Read the model definition and answer for the solid it produces. Units are mm, in the model's axes. Face numbers are marked on the shaded views. A direction names the side the tool comes from. Round coordinates to 2 decimals unless told otherwise and drop trailing zeros. Write each loop counter-clockwise with the first axis right and the second up, starting at its lowest first coordinate (ties: lowest second). Pieces come first, ordered by that corner, then holes. Notation, with made-up numbers: (79, 73) - (135, 73) arc R11 ccw to (135, 79) - close; hole circle Ø1 at (-34, 34). An arc over 180 degrees is marked (long way). Use one line per item in the form item = value. Start each with the question number.
1) For a pull along Z with two mould halves and no side action, classify the marked faces 1, 2 and 3 as released by +Z, released by -Z, zero draft, split by the parting line, or undercut.
2) The part is cut by section B-B, the plane x = -5.5. Give the vertices of the cut face in (y, z), plus the area to 3 significant figures.
3) The part is cut by section C-C, the plane y = -5.25. Count the separate pieces of the cut face and the enclosed holes in it, plus the area to 3 significant figures.
4) The part is cut by section A-A, the plane y = 7.25. Give the vertices of the cut face in (x, z).
5) Each of these flat-tipped pins is pushed along its axis until it touches: pin 1 (1.9 mm diameter, centred on y = -7.4, z = 4.28, fed in from +X); pin 2 (5 mm diameter, centred on x = -1.5, y = -3.5, fed in from -Z); pin 3 (3 mm diameter, centred on x = -12, z = 1, fed in from +Y). Where does it stop, or does it pass through?
6) Consider line 1 along X through (y, z) = (4.75, 2); line 2 along X through (y, z) = (-5.75, 1); line 3 along Y through (x, z) = (-4.25, -2.5). Determine where each line is inside the solid, lowest interval first. Write a range as from..to.
7) For the marked faces 4, 5, 6 and 7, determine the directions among +Z, -Z, +X, -X, +Y, -Y from which every point of the face is accessible in a straight line to the end or side of a thin tool.
from build123d import *

# Parameters (mm, degrees)
F4_DEPTH = 1.3
F6_DEPTH = 1.05
F5_R     = 0.725
F7_DEPTH = 0.67
F8_R     = 0.3621320344
F8_2_R   = 0.3621320344


# Not quite as in the source:
# - a fillet or chamfer that OpenCascade refuses, or shapes differently, is made with other operations: its cross-section is extruded or revolved along the edge and cut away or added


with BuildPart() as f1:
    # F0 (on Front) → F1 (revolve)
    with BuildSketch(Plane.XZ):
        Polygon((-8.85, 2), (-8.85, 0.75), (-2.35, 0.75), (-2.35, 6.5), (-7.85, 6.5), (-7.85, 2), align=None)
    revolve(axis=Axis((6.5496404592, 0, 0), (1, 0, 0)))

    # F3: chamfer of 2 x 1 on 1 edges, made by hand

    # F3_s1 → F3_t2 (revolve, cut)
    with BuildSketch(Plane.XZ):
        Polygon((-6.85, 6.5), (-7.85, 4.5), (-7.85, 6.5), align=None)
    revolve(axis=Axis((-7.85, 0, 0), (1, 0, 0)), mode=Mode.SUBTRACT)

    # F2 (on face) → F4 (cut)
    with BuildSketch(Plane(origin=(-7.85, 0, 0), x_dir=(0, -1, 0), z_dir=(-1, 0, 0))):
        with BuildLine():
            Line((-1.65, 2.2843407316), (-1.65, 6.2870899469))
            ThreePointArc((-1.65, 6.2870899469), (-5.6291651246, 3.25), (-6.2697796099, -1.7146030572))
            Line((-6.2697796099, -1.7146030572), (-2.8032971045, 0.2867715504))
            ThreePointArc((-2.8032971045, 0.2867715504), (-1.9590250278, 1.1310436271), (-1.65, 2.2843407316))
        make_face()
        with BuildLine():
            ThreePointArc((6.5, 0), (5.14660082, 3.9702015062), (1.65, 6.2870899469))
            Line((1.65, 6.2870899469), (1.65, 2.2843407316))
            ThreePointArc((1.65, 2.2843407316), (1.9590250278, 1.1310436271), (2.8032971045, 0.2867715504))
            Line((2.8032971045, 0.2867715504), (6.2697796099, -1.7146030572))
            ThreePointArc((6.2697796099, -1.7146030572), (6.4421878063, -0.8649949526), (6.5, 0))
        make_face()
        with BuildLine():
            Line((-1.1532971045, -2.571112282), (-4.6197796099, -4.5724868897))
            ThreePointArc((-4.6197796099, -4.5724868897), (0, -6.5), (4.6197796099, -4.5724868897))
            Line((4.6197796099, -4.5724868897), (1.1532971045, -2.571112282))
            ThreePointArc((1.1532971045, -2.571112282), (0, -2.2620872543), (-1.1532971045, -2.571112282))
        make_face()
    extrude(amount=-F4_DEPTH, mode=Mode.SUBTRACT)

    # F8
    f8_edges = [f1.edges().sort_by_distance(p)[0] for p in [
        (-7.85, 0, 4.5),
        (-7.85, 3.897114, -2.25),
        (-7.85, -3.897114, -2.25),
        (-8.85, 0, -2),
    ]]
    fillet(f8_edges, radius=F8_R)



with BuildPart() as f1b:
    # F0 (on Front) → F1, piece 2 (revolve)
    with BuildSketch(Plane.XZ):
        Polygon((-0.67, 0.75), (0, 0.75), (0, 6.2), (-1.05, 6.2), (-1.55, 6.5), (-2.05, 6.5), (-2.05, 5.64), (-0.67, 5.64), align=None)
    revolve(axis=Axis((6.5496404592, 0, 0), (1, 0, 0)))

    # F5 (on face) → F6 (cut)
    with BuildSketch(Plane.YZ):
        with BuildLine():
            ThreePointArc((4.3433258161, 4.4244232228), (0, 6.2), (-4.3433258161, 4.4244232228))
            Line((-4.3433258161, 4.4244232228), (-1.1869283577, 2.6020763005))
            ThreePointArc((-1.1869283577, 2.6020763005), (0, 2.86), (1.1869283577, 2.6020763005))
            Line((1.1869283577, 2.6020763005), (4.3433258161, 4.4244232228))
        make_face()
        with BuildLine():
            Line((1.66, -2.3289482605), (1.66, -5.9736421051))
            ThreePointArc((1.66, -5.9736421051), (4.936192865, -3.75153302), (6.2, 0))
            ThreePointArc((6.2, 0), (6.150634929, 0.780826466), (6.0033258161, 1.5492188823))
            Line((6.0033258161, 1.5492188823), (2.8469283577, -0.27312804))
            ThreePointArc((2.8469283577, -0.27312804), (2.4768326548, -1.43), (1.66, -2.3289482605))
        make_face()
        with BuildLine():
            ThreePointArc((-6.0033258161, 1.5492188823), (-5.3693575035, -3.1), (-1.66, -5.9736421051))
            Line((-1.66, -5.9736421051), (-1.66, -2.3289482605))
            ThreePointArc((-1.66, -2.3289482605), (-2.4768326548, -1.43), (-2.8469283577, -0.27312804))
            Line((-2.8469283577, -0.27312804), (-6.0033258161, 1.5492188823))
        make_face()
    extrude(amount=-F6_DEPTH, mode=Mode.SUBTRACT)

    # F5 (on face) → F7 (join)
    with BuildSketch(Plane.YZ):
        with BuildLine():
            Line((-8.2345172024, 2.8373978297), (-6.0033258161, 1.5492188823))
            ThreePointArc((-6.0033258161, 1.5492188823), (-5.3693575035, 3.1), (-4.3433258161, 4.4244232228))
            Line((-4.3433258161, 4.4244232228), (-6.5745172024, 5.7126021703))
            ThreePointArc((-6.5745172024, 5.7126021703), (-8.8421193726, 5.105), (-8.2345172024, 2.8373978297))
        make_face()
        with Locations((-7.4045172024, 4.275)):
            Circle(F5_R, mode=Mode.SUBTRACT)
        with BuildLine():
            ThreePointArc((4.3433258161, 4.4244232228), (5.3693575035, 3.1), (6.0033258161, 1.5492188823))
            Line((6.0033258161, 1.5492188823), (8.2345172024, 2.8373978297))
            ThreePointArc((8.2345172024, 2.8373978297), (8.8421193726, 5.105), (6.5745172024, 5.7126021703))
            Line((6.5745172024, 5.7126021703), (4.3433258161, 4.4244232228))
        make_face()
        with Locations((7.4045172024, 4.275)):
            Circle(F5_R, mode=Mode.SUBTRACT)
        with BuildLine():
            Line((1.66, -8.55), (1.66, -5.9736421051))
            ThreePointArc((1.66, -5.9736421051), (0, -6.2), (-1.66, -5.9736421051))
            Line((-1.66, -5.9736421051), (-1.66, -8.55))
            ThreePointArc((-1.66, -8.55), (0, -10.21), (1.66, -8.55))
        make_face()
        with Locations((0, -8.55)):
            Circle(F5_R, mode=Mode.SUBTRACT)
    extrude(amount=-F7_DEPTH)

    # F8#2
    f8_2_edges = [f1b.edges().sort_by_distance(p)[0] for p in [
        (-1.05, -5.750678, 1.403352),
        (-1.05, -4.090678, 4.278557),
        (-1.05, 4.090678, 4.278557),
        (-1.05, 5.750678, 1.403352),
        (-1.05, 1.66, -5.681909),
        (-1.05, -1.66, -5.681909),
    ]]
    fillet(f8_2_edges, radius=F8_2_R)

    # F9: chamfer of 2.2 x 0.5 on 1 edges, made by hand

    # F9_s1 → F9_t2 (revolve, cut)
    with BuildSketch(Plane.XZ):
        Polygon((0, 2.95), (-0.5, 0.75), (0, 0.75), align=None)
    revolve(axis=Axis((0, 0, 0), (1, 0, 0)), mode=Mode.SUBTRACT)


with BuildPart() as f1_1:
    add(f1.part)

    add(f1b.part)  # F10 merges F1b
    # F0 (on Front) → F10 (revolve)
    with BuildSketch(Plane.XZ):
        Polygon((-14.92, 0.75), (-14.92, 0), (0.62, 0), (0.62, 0.75), (0, 0.75), (-0.67, 0.75), (-2.35, 0.75), (-8.85, 0.75), align=None)
    revolve(axis=Axis((6.5496404592, 0, 0), (1, 0, 0)))


solid = f1_1.part
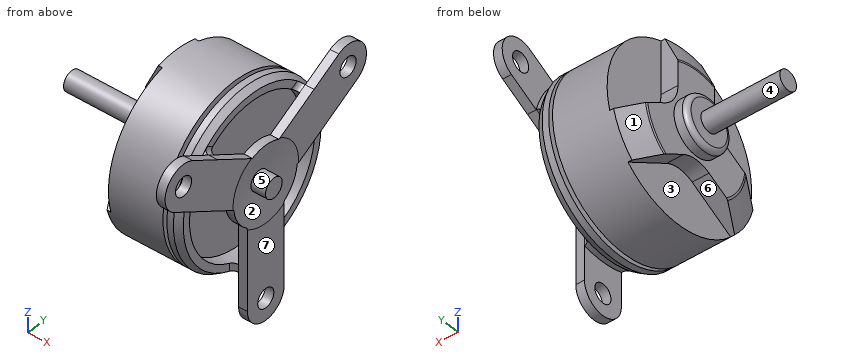
Geometry results:
q1.face_1 = released by -Z
q1.face_2 = undercut
q1.face_3 = zero draft
q2.outline = circle Ø13 at (0, 0)
q2.area = 133 mm2
q3.separate_pieces = 3
q3.enclosed_holes = 0
q3.area = 40.2 mm2
q4.outline = (-0.67, 2.27) - (0, 2.27) - (0, 3.57) - (-0.67, 3.57) - close; (-0.67, 4.98) - (0, 4.98) - (0, 5.93) - (-0.67, 5.93) - close
q5.pin_1 = 0
q5.pin_2 = -9.75
q5.pin_3 = 0.75
q6.line_1 = -6.55..-2.35, -0.67..0
q6.line_2 = -6.55..-2.35, -2.05..-1.05
q6.line_3 = -6..6
q7.face_4 = -X
q7.face_5 = +X
q7.face_6 = -Z, -X
q7.face_7 = -Z, +X, +Y, -Y
